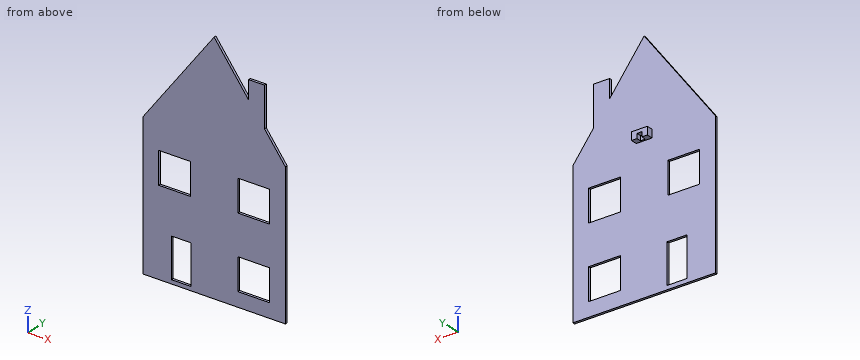
```python
from build123d import *

# Parameters (mm, degrees)
F0_W     = 900
F0_H     = 900
F0_W_2   = 125
F0_H_2   = 250
F0_W_3   = 200
F0_H_3   = 200
F1_DEPTH = 15
F3_DEPTH = 40
F4_W     = 30
F4_H     = 30
F5_DEPTH = 30


with BuildPart() as f1:
    # F0 (on Front) → F1 (new body)
    with BuildSketch(Plane.XZ):
        with Locations((-68.50922, -158.423999)):
            Rectangle(F0_W, F0_H)
        with Locations((-275.546044, -458.423999)):
            Rectangle(F0_W_2, F0_H_2, mode=Mode.SUBTRACT)
        with Locations((-318.50922, 31.576001)):
            Rectangle(F0_W_3, F0_H_3, mode=Mode.SUBTRACT)
        with Locations((181.49078, -418.423999)):
            Rectangle(F0_W_3, F0_H_3, mode=Mode.SUBTRACT)
        with Locations((181.49078, 31.576001)):
            Rectangle(F0_W_3, F0_H_3, mode=Mode.SUBTRACT)
        Polygon((-518.50922, 291.576001), (381.49078, 291.576001), (249.479083, 467.591597), (149.479083, 600.92493), (-68.50922, 891.576001), align=None)
        Polygon((149.479083, 600.92493), (249.479083, 467.591597), (249.479083, 717.591597), (149.479083, 717.591597), align=None)
    extrude(amount=F1_DEPTH)

    # F2 (on face) → F3 (join)
    with BuildSketch(Plane(origin=(0, 0, 0), x_dir=(-1, 0, 0), z_dir=(0, 1, 0))):
        Polygon((18.50922, 291.576001), (68.50922, 291.576001), (118.50922, 291.576001), (118.50922, 341.576001), (18.50922, 341.576001), align=None)
    extrude(amount=F3_DEPTH)

    # F4 (on face) → F5 (cut)
    with BuildSketch(Plane(origin=(0, 40, 0), x_dir=(-1, 0, 0), z_dir=(0, 1, 0))):
        with Locations((68.50922, 306.576001)):
            Rectangle(F4_W, F4_H)
    extrude(amount=-F5_DEPTH, mode=Mode.SUBTRACT)


solid = f1.part
```
Can you work these out from the model? Positions are in its coordinate system, mm. Round coordinates to 2 decimals unless told otherwise and drop trailing zeros. Loops run counter-clockwise (first coordinate to the right, second up) from the corner with the lowest first, then second, coordinate; pieces in that order, holes last. Notation, with made-up numbers: M 40,-31 L 87,-31 A20 cw 87,-12 Z; hole C 18,63 d11. An arc over 180 degrees is marked long. Write item = value, one per line. Start each with the question number.
(1) Suppose I cut it at C-C on y = 26. Write out the boundary of the cut face in (x, z).
(2) Suppose I cut it at D-D on x = -400. Write out the boundary of the cut face in (y, z), plus the area to 3 significant figures.
(3) Suppose I cut it at B-B on x = 182. Write out the boundary of the cut face in (y, z).
(4) I need wall thicknesses on line 1 along Z through (x, y) = (-251, -1); line 2 along Y through (x, z) = (-162, 508); line 3 along Z through (x, y) = (-97, 28.5). Which ranges of each line are inside material? Lowest first, please.
(5) I'm going to push flat-ended pins straight in: P1, Ø24, axis at y = 20.5, z = 312.5, coming from the -X side; P2, Ø16.5, axis at x = 213, y = -5, coming from the +Z side; P3, Ø8, axis at x = 34.5, z = -80, coming from the +Y side. Where does each tip first touch, or does it pass through?
(6) Suppose I cut it at A-A on z = -18. Write out the boundary of the cut face in (x, y), plus the area to 3 significant figures.
Answer block:
q1.outline = M -118.51,291.58 L -83.51,291.58 L -83.51,321.58 L -53.51,321.58 L -53.51,291.58 L -18.51,291.58 L -18.51,341.58 L -118.51,341.58 Z
q2.outline = M -15,-608.42 L 0,-608.42 L 0,-68.42 L -15,-68.42 Z; M -15,131.58 L 0,131.58 L 0,449.59 L -15,449.59 Z
q2.area = 12,900 mm²
q3.outline = M -15,-608.42 L 0,-608.42 L 0,-518.42 L -15,-518.42 Z; M -15,-318.42 L 0,-318.42 L 0,-68.42 L -15,-68.42 Z; M -15,131.58 L 0,131.58 L 0,717.59 L -15,717.59 Z
q4.line_1 = -608.42 to -583.42, -333.42 to -68.42, 131.58 to 648.25
q4.line_2 = -15 to 0
q4.line_3 = 291.58 to 341.58
q5.P1 = -118.51
q5.P2 = 717.59
q5.P3 = 0
q6.outline = M -518.51,-15 L -418.51,-15 L -418.51,0 L -518.51,0 Z; M -218.51,-15 L 81.49,-15 L 81.49,0 L -218.51,0 Z; M 281.49,-15 L 381.49,-15 L 381.49,0 L 281.49,0 Z
q6.area = 7,500 mm²
